For this review, take the finished solid that the model builds, in its own axes (mm). Round coordinates to 2 decimals unless told otherwise and drop trailing zeros. Loops run counter-clockwise (first coordinate to the right, second up) from the corner with the lowest first, then second, coordinate; pieces in that order, holes last. Notation, with made-up numbers: (11.25, 33) -> (61.25, 33) arc R29 cw to (61.25, 57) -> close; hole circle Ø11 at (64, -14). An arc over 180 degrees is marked (long way). Write each question's results on one line, items separated by ' | '.
```python
from build123d import *

# Parameters (mm, degrees)
F0_R     = 11
F1_DEPTH = 3


with BuildPart() as f1:
    # F0 (on Top) → F1 (new body)
    with BuildSketch(Plane.XY):
        with BuildLine():
            ThreePointArc((-4.80491, 33.996037), (-11.97758, 22.266799), (-3.427827, 11.5))
            ThreePointArc((-3.427827, 11.5), (-12, 0), (-3.427827, -11.5))
            ThreePointArc((-3.427827, -11.5), (-11.97758, -22.266799), (-4.80491, -33.996037))
            Line((-4.80491, -33.996037), (0, -39.177649))
            Line((0, -39.177649), (4.80491, -33.996037))
            ThreePointArc((4.80491, -33.996037), (11.97758, -22.266799), (3.427827, -11.5))
            ThreePointArc((3.427827, -11.5), (12, 0), (3.427827, 11.5))
            ThreePointArc((3.427827, 11.5), (11.97758, 22.266799), (4.80491, 33.996037))
            Line((4.80491, 33.996037), (0, 39.177649))
            Line((0, 39.177649), (-4.80491, 33.996037))
        make_face()
        with Locations((0, -23)):
            Circle(F0_R, mode=Mode.SUBTRACT)
        Circle(F0_R, mode=Mode.SUBTRACT)
        with Locations((0, 23)):
            Circle(F0_R, mode=Mode.SUBTRACT)
    extrude(amount=F1_DEPTH)


solid = f1.part
```
1. For pin 1 (1 mm diameter, centred on x = -1.5, z = 2.5, fed in from +Y); pin 2 (6 mm diameter, centred on x = 7, y = 0.5, fed in from +Z), all flat-tipped, find the tip position at first contact; note any pin that passes through.
Values found:
pin 1: stops at y = 38.1 | pin 2: passes through
2. Consider section A-A (y = 23). State the section outline as (x, z) points, plus the area to 3 significant figures.
Values found:
outline: (-12, 0) -> (-11, 0) -> (-11, 3) -> (-12, 3) -> close; (11, 0) -> (12, 0) -> (12, 3) -> (11, 3) -> close | area: 6.00 mm2
3. To check wall thickness, follow probe 1 along Y at (x, z) = (7.25, 1.5); probe 2 along Y at (x, z) = (10, 1.4); probe 3 along X at (y, z) = (16.5, 1). State the ranges of each line that lie inside material, in increasing order.
Values found:
probe 1: y = -32.56 to -31.27, -14.73 to -13.44, -9.56 to -8.27, 8.27 to 9.56, 13.44 to 14.73, 31.27 to 32.56 | probe 2: y = -29.63 to -27.58, -18.42 to -16.37, -6.63 to -4.58, 4.58 to 6.63, 16.37 to 18.42, 27.58 to 29.63 | probe 3: x = -10.09 to -8.87, 8.87 to 10.09
4. Draft analysis for pull direction Y (two halves, no side actions). For faces 1 (the face through (2.37, -36.62, 1.48)), 2 (the face through (-2.38, -33.74, 1.48)), 3 (the face through (-7, -9, 0)), state which applies: released by +Y, released by -Y, zero draft, split by the parting line, or undercut.
Values found:
face 1: released by -Y | face 2: undercut | face 3: zero draft
5. Consider section B-B (z = 1.45). State the section outline as (x, y) points, plus the area to 3 significant figures.
Values found:
outline: (-4.8, -34) -> (0, -39.18) -> (4.8, -34) arc R12 ccw to (3.43, -11.5) arc R12 ccw to (3.43, 11.5) arc R12 ccw to (4.8, 34) -> (0, 39.18) -> (-4.8, 34) arc R12 ccw to (-3.43, 11.5) arc R12 ccw to (-3.43, -11.5) arc R12 ccw to start; hole circle Ø22 at (0, -23); hole circle Ø22 at (0, 0); hole circle Ø22 at (0, 23) | area: 244 mm2
6. Consider section C-C (x = 10). State the section outline as (y, z) points, plus the area to 3 significant figures.
Values found:
outline: (-29.63, 0) -> (-27.58, 0) -> (-27.58, 3) -> (-29.63, 3) -> close; (-18.42, 0) -> (-16.37, 0) -> (-16.37, 3) -> (-18.42, 3) -> close; (-6.63, 0) -> (-4.58, 0) -> (-4.58, 3) -> (-6.63, 3) -> close; (4.58, 0) -> (6.63, 0) -> (6.63, 3) -> (4.58, 3) -> close; (16.37, 0) -> (18.42, 0) -> (18.42, 3) -> (16.37, 3) -> close; (27.58, 0) -> (29.63, 0) -> (29.63, 3) -> (27.58, 3) -> close | area: 36.9 mm2
7. Consider section D-D (y = -29.5). State the section outline as (x, z) points.
Values found:
outline: (-10.09, 0) -> (-8.87, 0) -> (-8.87, 3) -> (-10.09, 3) -> close; (8.87, 0) -> (10.09, 0) -> (10.09, 3) -> (8.87, 3) -> close
